```python
from build123d import *

# Parameters (mm, degrees)
SKETCH_194_W       = 23.879073069
SKETCH_194_H       = 2
SKETCH_194_W_2     = 13.873866224
SKETCH_194_H_2     = 3.944574251
SKETCH_194_R       = 2.25
EXTRUDE_1_DEPTH    = 2
SKETCH_2_W         = 8
SKETCH_2_H         = 2
EXTRUDE_3672_DEPTH = 2


with BuildPart() as part:
    # Sketch 194 → 凸台-拉伸1 (new body)
    with BuildSketch(Plane(origin=(0, 0, 0), x_dir=(0, 0, -1), z_dir=(1, 0, 0))):
        with BuildLine():
            Line((-95.202576637, 16.678130112), (-96.66172395, 0))
            Line((-96.66172395, 0), (-44.182229478, 0))
            ThreePointArc((-44.182229478, 0), (-41.932229478, 2.25), (-39.682229478, 0))
            Line((-39.682229478, 0), (-23.132229478, 0))
            ThreePointArc((-23.132229478, 0), (-20.882229478, 2.25), (-18.632229478, 0))
            Line((-18.632229478, 0), (38.58827605, 0))
            Line((38.58827605, 0), (38.58827605, 4.627371722))
            Line((38.58827605, 4.627371722), (53.708180549, 16.713080595))
            Line((53.708180549, 16.713080595), (53.708180549, 19.964535026))
            Line((53.708180549, 19.964535026), (49.47062371, 25.265958003))
            ThreePointArc((49.47062371, 25.265958003), (48.71615842, 24.206772475), (47.878069959, 23.212438733))
            Line((47.878069959, 23.212438733), (45.32875497, 25.545040291))
            ThreePointArc((45.32875497, 25.545040291), (46.329625978, 26.78976103), (47.163951689, 28.151735001))
            Line((47.163951689, 28.151735001), (38.58827605, 38.88038965))
            Line((38.58827605, 38.88038965), (37.693344157, 40))
            Line((37.693344157, 40), (-18.632229478, 40))
            ThreePointArc((-18.632229478, 40), (-20.882229478, 37.75), (-23.132229478, 40))
            Line((-23.132229478, 40), (-39.682229478, 40))
            ThreePointArc((-39.682229478, 40), (-41.932229478, 37.75), (-44.182229478, 40))
            Line((-44.182229478, 40), (-87.664190365, 40))
            ThreePointArc((-87.664190365, 40), (-91.717731611, 38.423664021), (-93.641358554, 34.522934456))
            Line((-93.641358554, 34.522934456), (-94.87665585, 20.403421746))
            ThreePointArc((-94.87665585, 20.403421746), (-92.775563539, 19.482408503), (-90.560913042, 18.883929203))
            Line((-90.560913042, 18.883929203), (-91.219638908, 15.446476624))
            ThreePointArc((-91.219638908, 15.446476624), (-93.245188063, 15.952094064), (-95.202576637, 16.678130112))
        make_face()
        with Locations((-32.321766012, 13.338077)):
            Rectangle(SKETCH_194_W, SKETCH_194_H, mode=Mode.SUBTRACT)
        with Locations((-32.321766012, 17.395875517)):
            Rectangle(SKETCH_194_W, SKETCH_194_H, mode=Mode.SUBTRACT)
        with Locations((-12.198657062, 12.527713279)):
            Rectangle(SKETCH_194_W_2, SKETCH_194_H_2, mode=Mode.SUBTRACT)
        with BuildLine():
            ThreePointArc((-68.122104991, 24.366829507), (-68.414052328, 21.766100622), (-71.014781213, 22.058047959))
            Line((-71.014781213, 22.058047959), (-79.877790346, 33.162526768))
            ThreePointArc((-79.877790346, 33.162526768), (-79.585843009, 35.763255653), (-76.985114123, 35.471308316))
            Line((-76.985114123, 35.471308316), (-68.122104991, 24.366829507))
        make_face(mode=Mode.SUBTRACT)
        with BuildLine():
            ThreePointArc((-58.122104991, 24.366829507), (-58.414052328, 21.766100622), (-61.014781213, 22.058047959))
            Line((-61.014781213, 22.058047959), (-69.877790346, 33.162526768))
            ThreePointArc((-69.877790346, 33.162526768), (-69.585843009, 35.763255653), (-66.985114123, 35.471308316))
            Line((-66.985114123, 35.471308316), (-58.122104991, 24.366829507))
        make_face(mode=Mode.SUBTRACT)
        with BuildLine():
            ThreePointArc((-48.122104991, 24.366829507), (-48.414052328, 21.766100622), (-51.014781213, 22.058047959))
            Line((-51.014781213, 22.058047959), (-59.877790346, 33.162526768))
            ThreePointArc((-59.877790346, 33.162526768), (-59.585843009, 35.763255653), (-56.985114123, 35.471308316))
            Line((-56.985114123, 35.471308316), (-48.122104991, 24.366829507))
        make_face(mode=Mode.SUBTRACT)
        with Locations((-87.664190365, 34)):
            Circle(SKETCH_194_R, mode=Mode.SUBTRACT)
        with Locations((36.08827605, 34)):
            Circle(SKETCH_194_R, mode=Mode.SUBTRACT)
    extrude(amount=EXTRUDE_1_DEPTH)

    # 草图2 → Extrude 3672 (add)
    with BuildSketch(Plane(origin=(0, 0, 0), x_dir=(0, 0, -1), z_dir=(1, 0, 0))):
        with Locations((31.58827605, -1)):
            Rectangle(SKETCH_2_W, SKETCH_2_H)
        with BuildLine():
            Line((-83.862737476, 52.5), (-85.358986401, 42))
            ThreePointArc((-85.358986401, 42), (-86.138250874, 40.569690448), (-87.664190365, 40))
            Line((-87.664190365, 40), (-65.306655843, 40))
            Line((-65.306655843, 40), (-57.306655843, 40))
            Line((-57.306655843, 40), (-57.306655843, 42))
            Line((-57.306655843, 42), (-65.306655843, 42))
            Line((-65.306655843, 42), (-75.139107316, 52.5))
            Line((-75.139107316, 52.5), (-83.862737476, 52.5))
        make_face()
        with Locations((1.58827605, -1)):
            Rectangle(SKETCH_2_W, SKETCH_2_H)
        with Locations((-58.41172395, -1)):
            Rectangle(SKETCH_2_W, SKETCH_2_H)
        with Locations((-88.41172395, -1)):
            Rectangle(SKETCH_2_W, SKETCH_2_H)
        with Locations((28.693344157, 41)):
            Rectangle(SKETCH_2_W, SKETCH_2_H)
        with Locations((-1.306655843, 41)):
            Rectangle(SKETCH_2_W, SKETCH_2_H)
        with Locations((-31.306655843, 41)):
            Rectangle(SKETCH_2_W, SKETCH_2_H)
    extrude(amount=EXTRUDE_3672_DEPTH)


solid = part.part
```
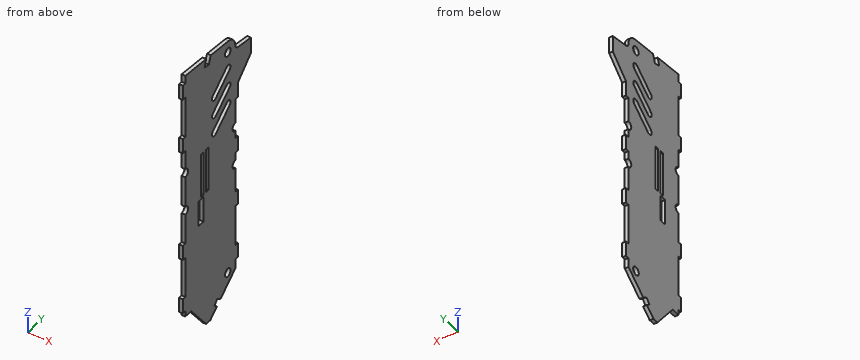
Model file for the job. Use its own axes, mm. Coordinates: 2 decimals unless noted, no trailing zeros. Loops run counter-clockwise (first coordinate to the right, second up) from the corner with the lowest first, then second, coordinate; pieces in that order, holes last. Notation, with made-up numbers: (-16, 46.5) - (10, 46.5) arc R27 cw to (10, 71.5) - close; hole circle Ø10 at (84, 76.25). An arc over 180 degrees is marked (long way). Answer as a JSON object with one key per item and string values. Group by question number.
(1) Flat gauge pins, fed straight in: pin 1 (0.6 mm diameter, centred on x = 1, y = 41, fed in from +Z); pin 2 (1 mm diameter, centred on x = 0.5, z = 35, fed in from +Y); pin 3 (1 mm diameter, centred on x = 1, y = 41, fed in from -Z). Where does each tip first touch, or does it go through?
(2) Cut at C-C (y = 45). Give the cut face in (x, z).
(3) Cut at D-D (z = -42). Give the cut face in (x, y), then the cut area to 3 significant figures.
(4) Cut at A-A (z = 7). Give the cut face in (x, y), then the cut area to 3 significant figures.
(5) Cut at B-B (x = 1). State how many separate pieces and enclosed holes the cut face has, then the cut area to 3 significant figures.
(6) Probe line 1 along Y through (x, z) = (0.15, 21); line 2 along Y through (x, z) = (0.3, 24.5); line 3 along Z through (x, y) = (1.15, 22). List the from-to ranges inside material, lowest first.
Geometry says:
{
 "1": {"pin 1": "stops at z = 86", "pin 2": "stops at y = 42", "pin 3": "stops at z = -32.69"},
 "2": {"outline": "(0, 68.12) - (2, 68.12) - (2, 84.93) - (0, 84.93) - close"},
 "3": {"outline": "(0, 7.35) - (2, 7.35) - (2, 34.61) - (0, 34.61) - close", "area": "54.5 mm^2"},
 "4": {"outline": "(0, 0) - (2, 0) - (2, 10.56) - (0, 10.56) - close; (0, 14.5) - (2, 14.5) - (2, 40) - (0, 40) - close", "area": "72.1 mm^2"},
 "5": {"separate pieces": "1", "enclosed holes": "8", "area": "5,510 mm^2"},
 "6": {"line 1": "y = 2.25 to 12.34, 14.34 to 16.4, 18.4 to 37.75", "line 2": "y = 0 to 12.34, 14.34 to 16.4, 18.4 to 40", "line 3": "z = -52.08 to 48.17, 50.97 to 58.17, 60.97 to 68.17, 70.97 to 94.74"}
}
